Job drawing, mm, ordinate dimensions from the low corner. One solid piece. A direction names the side the tool comes from. Round coordinates to 2 decimals unless told otherwise and drop trailing zeros. Loops run counter-clockwise (first coordinate to the right, second up) from the corner with the lowest first, then second, coordinate; pieces in that order, holes last. Notation, with made-up numbers: M -27,57.25 L 31,57.25 A35 cw 31,93.25 Z; hole C 20,-16.5 d9. An arc over 180 degrees is marked long. Put each result on its own line as item: value. Start each with the question number.
1) Slice it at B-B on z = 18. Give the cut face in (x, y), then the cut area to 3 significant figures.
2) Probe line 1 along X through (y, z) = (22.5, 5); line 2 along Y through (x, z) = (60, 22.5). List the from-to ranges inside material, lowest first.
3) Pull direction Z, two halves, no side cores. Call the marked faces 1, 2 and 3: +Z half, -Z half, draft (parallel to the pull), parting line (faces both ways), or undercut.
4) Drop a flat-ended pin along its axis: pin 1 Ø19.5 at (x, z) = (36, 40) entering from +Y. Give the stop position or say it passes through.
5) Which spindle directions (+Z, -Z, +X, -X, +Y, -Y) get a long thin tool onto all of the face, cutting with end or side? Do the marked faces 4 and 5. Say none if no direction does.
6) Slice it at C-C on y = 6.5. Give the cut face in (x, z), then the cut area to 3 significant figures.
7) Slice it at D-D on x = 61. Give the cut face in (y, z), then the cut area to 3 significant figures.
8) Slice it at A-A on y = 14. Give the cut face in (x, z), then the cut area to 3 significant figures.
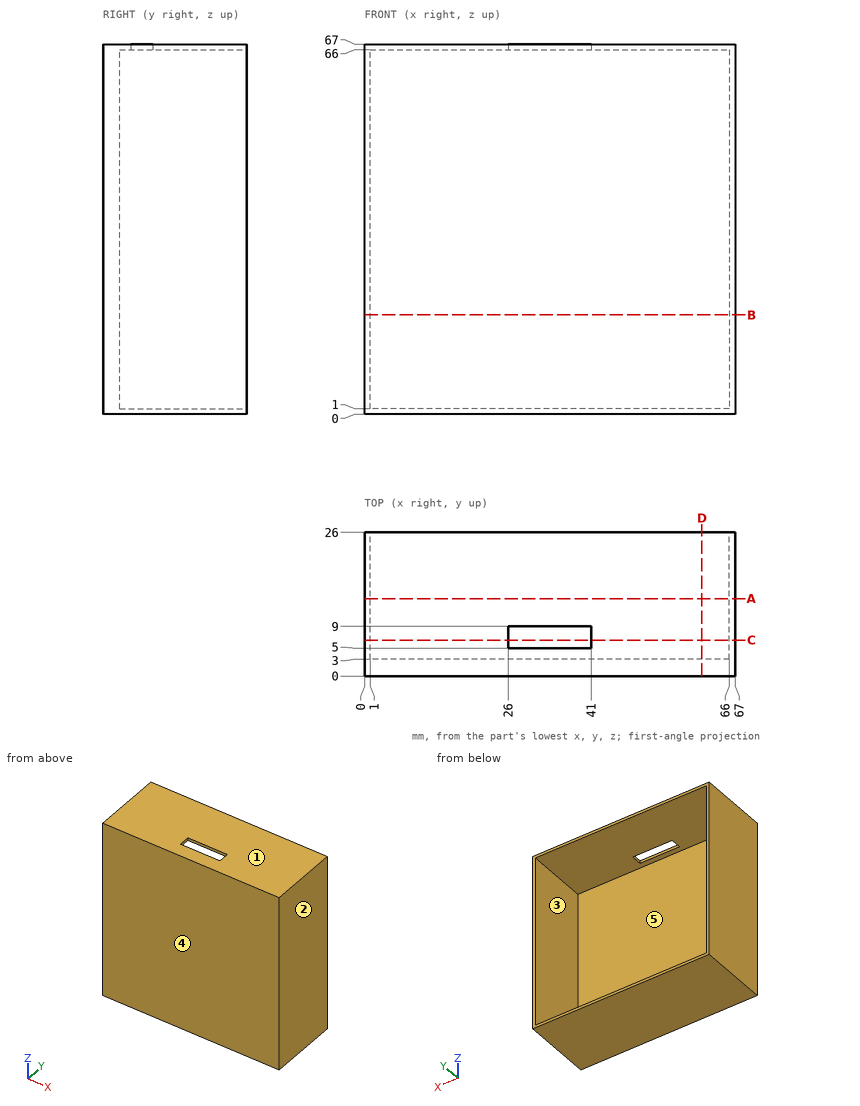
Recorded:
1. outline: M 0,0 L 67,0 L 67,26 L 66,26 L 66,3 L 1,3 L 1,26 L 0,26 Z
1. area: 247 mm2
2. line 1: x = 0 to 1, 66 to 67
2. line 2: y = 0 to 3
3. face 1: +Z half
3. face 2: draft
3. face 3: undercut
4. pin 1: stops at y = 3
5. face 4: +Z, -Z, +X, -X, -Y
5. face 5: +Y
6. outline: M 0,0 L 67,0 L 67,67 L 41,67 L 41,66 L 66,66 L 66,1 L 1,1 L 1,66 L 26,66 L 26,67 L 0,67 Z
6. area: 249 mm2
7. outline: M 0,0 L 26,0 L 26,1 L 3,1 L 3,66 L 26,66 L 26,67 L 0,67 Z
7. area: 247 mm2
8. outline: M 0,0 L 67,0 L 67,67 L 0,67 Z; hole M 1,1 L 66,1 L 66,66 L 1,66 Z
8. area: 264 mm2
